Geometry: final body of the model. Coordinates: model frame, mm. A direction names the side the tool comes from. Give positions to 0.01 mm unless a question says otherwise; leave off trailing zeros. Write each loop counter-clockwise with the first axis right and the second up, starting at its lowest first coordinate (ties: lowest second). Pieces come first, ordered by that corner, then holes. Notation, with made-up numbers: M 24.25,-3.75 L 57.25,-3.75 A13 cw 57.25,11.25 Z; hole C 23.5,3 d9. An arc over 180 degrees is marked long. Use a Markdown table: item, result. Add a question column.
(1) Draft query along X for faces 1 (the flat face through (112, 84, 25)), 2 (the flat face through (54, 0, 25)), 3 (the flat face through (54, 86, -2)). Return one class per face: released by +X, released by -X, zero draft, split by the parting line, or undercut.
(2) Cut plane A-A (y = 70). Output: boundary loops of the cut face in (x, z), plus the area to 3 significant figures.
(3) Cut plane B-B (x = 13.5). Output: boundary loops of the cut face in (y, z), plus the area to 3 significant figures.
(4) Cut plane C-C (z = 11). Output: boundary loops of the cut face in (x, y), plus the area to 3 significant figures.
(5) Reachability of faces 4 (the flat face through (0, 84, 25)), 5 (the cylindrical face through (110.378, 26.419, 31.548)), 6 (the cylindrical face through (24.54, -0.38, 27.95)) from +Z, -Z, +X, -X, +Y, -Y: full face, straight path, thin tool, end or side. Return the list, or none.
(6) Pin query (flat end, axial travel): pin 1 Ø3 at (x, y) = (4.5, 8) entering from -Z; pin 2 Ø7.5 at (x, y) = (80.5, 142.5) entering from +Z; pin 3 Ø4 at (x, y) = (66, 149.5) entering from +Z; pin 4 Ø3.5 at (y, z) = (110, 30) entering from +X. Return the tip coordinate at first contact, or that it passes through.
(7) Material intervals for L1, parallel to X at y = 143, z = 0.5; L2, parallel to Y at x = 70, z = 16; L3, parallel to X at y = 159, z = 24.5, sorted ascending.
(8) Cut plane D-D (y = 25). Output: boundary loops of the cut face in (x, z).
```python
from build123d import *

# Parameters (mm, degrees)
CYLINDER002_R            = 2.1
CYLINDER002_DEPTH        = 10
CYLINDER002_PITCH_ANGLE  = 90
CYLINDER001_R            = 1.6
CYLINDER001_DEPTH        = 7
ARRAY001_X_COUNT         = 2
ARRAY001_X_PITCH         = 76
ARRAY001_Y_COUNT         = 2
ARRAY001_Y_PITCH         = 135
CLONE003_ROLL_ANGLE      = 90
CLONE003_PLACEMENT_ANGLE = -90
CYLINDER_R               = 3.5
CYLINDER_DEPTH           = 3.5
ARRAY_X_COUNT            = 2
ARRAY_X_PITCH            = 76
ARRAY_Y_COUNT            = 2
ARRAY_Y_PITCH            = 135
CONE_PITCH_ANGLE         = -90
CLONE002_ROLL_ANGLE      = -90
CLONE002_PLACEMENT_ANGLE = -90
BOX_W                    = 110
BOX_H                    = 170
BOX_DEPTH                = 50
THICKNESS_T              = 2


with BuildPart() as cylinder002:
    # Cylinder002 → Cylinder002 (new body)
    with BuildSketch(Plane.XY):
        Circle(CYLINDER002_R)
    extrude(amount=CYLINDER002_DEPTH)


with BuildPart() as cylinder002_1:
    # Cylinder002 pitch: moved
    add(cylinder002.part.rotate(Axis((0, 0, 0), (0, 1, 0)), CYLINDER002_PITCH_ANGLE))


with BuildPart() as cylinder002_2:
    # Cylinder002 placement: moved
    add(cylinder002_1.part.moved(Location((108, 25, 30))))


with BuildPart() as clone_of_cylinder002:
    # Clone001 base: copy of Cylinder002
    add(cylinder002_2.part)


with BuildPart() as clone_of_cylinder002_1:
    # Clone001 placement: moved
    add(clone_of_cylinder002.part.moved(Location((0, 85, 0))))


with BuildPart() as mount_holes:
    # Cylinder001 → Cylinder001 (new body)
    with BuildSketch(Plane.XY.offset(-3)):
        Circle(CYLINDER001_R)
    extrude(amount=CYLINDER001_DEPTH)

    # Array001 X: mount_holes ×2


with BuildPart() as mount_holes_1:
    add(mount_holes.part)
    with Locations(*[(i * ARRAY001_X_PITCH, 0, 0) for i in range(1, ARRAY001_X_COUNT)]):
        add(mount_holes.part)

    # Array001 Y: mount_holes ×2


with BuildPart() as mount_holes_2:
    add(mount_holes_1.part)
    with Locations(*[(0, i * ARRAY001_Y_PITCH, 0) for i in range(1, ARRAY001_Y_COUNT)]):
        add(mount_holes_1.part)


with BuildPart() as mount_holes_3:
    # Array001 placement: moved
    add(mount_holes_2.part.moved(Location((4.5, 8, 0))))


with BuildPart() as fusion001:
    # Clone003 base: copy of Cylinder002
    add(cylinder002_2.part)


with BuildPart() as fusion001_1:
    # Clone003 roll: moved
    add(fusion001.part.rotate(Axis((0, 0, 0), (1, 0, 0)), CLONE003_ROLL_ANGLE))


with BuildPart() as fusion001_2:
    # Clone003 placement: moved
    add(fusion001_1.part.moved(Location((55, 113, 5))).rotate(Axis((55, 113, 5), (0, 0, 1)), CLONE003_PLACEMENT_ANGLE))

    # Fusion001: union Clone of Cylinder002, Cylinder002, mount_holes
    add(clone_of_cylinder002_1.part)
    add(cylinder002_2.part)
    add(mount_holes_3.part)


with BuildPart() as mount_points:
    # Cylinder → Cylinder (new body)
    with BuildSketch(Plane.XY):
        Circle(CYLINDER_R)
    extrude(amount=CYLINDER_DEPTH)

    # Array X: mount_points ×2


with BuildPart() as mount_points_1:
    add(mount_points.part)
    with Locations(*[(i * ARRAY_X_PITCH, 0, 0) for i in range(1, ARRAY_X_COUNT)]):
        add(mount_points.part)

    # Array Y: mount_points ×2


with BuildPart() as mount_points_2:
    add(mount_points_1.part)
    with Locations(*[(0, i * ARRAY_Y_PITCH, 0) for i in range(1, ARRAY_Y_COUNT)]):
        add(mount_points_1.part)


with BuildPart() as mount_points_3:
    # Array placement: moved
    add(mount_points_2.part.moved(Location((4.5, 8, 0))))


with BuildPart() as cone:
    # Cone → Cone (revolve)
    with BuildSketch(Plane.XZ):
        Polygon((0, 0), (8, 0), (4, 1.2), (0, 1.2), align=None)
    revolve(axis=Axis((0, 0, 0), (0, 0, 1)))


with BuildPart() as cone_1:
    # Cone pitch: moved
    add(cone.part.rotate(Axis((0, 0, 0), (0, 1, 0)), CONE_PITCH_ANGLE))


with BuildPart() as cone_2:
    # Cone placement: moved
    add(cone_1.part.moved(Location((110, 25, 30))))


with BuildPart() as clone_of_cone:
    # Clone base: copy of Cone
    add(cone_2.part)


with BuildPart() as clone_of_cone_1:
    # Clone placement: moved
    add(clone_of_cone.part.moved(Location((0, 85, 0))))


with BuildPart() as clone_of_cone001:
    # Clone002 base: copy of Cone
    add(cone_2.part)


with BuildPart() as clone_of_cone001_1:
    # Clone002 roll: moved
    add(clone_of_cone001.part.rotate(Axis((0, 0, 0), (1, 0, 0)), CLONE002_ROLL_ANGLE))


with BuildPart() as clone_of_cone001_2:
    # Clone002 placement: moved
    add(clone_of_cone001_1.part.moved(Location((-5, 110, 55))).rotate(Axis((-5, 110, 55), (0, 0, 1)), CLONE002_PLACEMENT_ANGLE))


with BuildPart() as case_with_mount_holes:
    # Box → Box (new body)
    with BuildSketch(Plane.XY):
        with Locations((55, 85)):
            Rectangle(BOX_W, BOX_H)
    extrude(amount=BOX_DEPTH)

    # Thickness
    thickness_openings = [case_with_mount_holes.faces().sort_by_distance(p)[0] for p in [
        (55, 85, 50),
    ]]
    offset(amount=THICKNESS_T, openings=thickness_openings)

    # Fusion: union mount_points, Clone of Cone, Cone, Clone of Cone001
    add(mount_points_3.part)
    add(clone_of_cone_1.part)
    add(cone_2.part)
    add(clone_of_cone001_2.part)

    # Cut: cut Fusion001
    add(fusion001_2.part, mode=Mode.SUBTRACT)


solid = case_with_mount_holes.part
```
Answer list:
| question | item | result |
|---|---|---|
| 1 | face 1 | released by +X |
| 1 | face 2 | undercut |
| 1 | face 3 | zero draft |
| 2 | outline | M -2,0 A2 ccw 0,-2 L 110,-2 A2 ccw 112,0 L 112,50 L 110,50 L 110,0 L 0,0 L 0,50 L -2,50 Z |
| 2 | area | 426 mm² |
| 3 | outline | M -2,0 A2 ccw 0,-2 L 170,-2 A2 ccw 172,0 L 172,50 L 170,50 L 170,0 L 0,0 L 0,50 L -2,50 Z |
| 3 | area | 546 mm² |
| 4 | outline | M -2,0 A2 ccw 0,-2 L 110,-2 A2 ccw 112,0 L 112,170 A2 ccw 110,172 L 0,172 A2 ccw -2,170 Z; hole M 0,0 L 110,0 L 110,170 L 0,170 Z |
| 4 | area | 1,130 mm² |
| 5 | face 4 | +Z |
| 5 | face 5 | +X |
| 5 | face 6 | -Y |
| 6 | pin 1 | through |
| 6 | pin 2 | z = 3.5 |
| 6 | pin 3 | z = 0 |
| 6 | pin 4 | x = 0 |
| 7 | L1 | -2 to 0, 1 to 2.9, 6.1 to 8, 77 to 78.9, 82.1 to 84, 110 to 112 |
| 7 | L2 | -2 to 0, 170 to 172 |
| 7 | L3 | -2 to 0, 110 to 112 |
| 8 | outline | M -2,0 A2 ccw 0,-2 L 110,-2 A2 ccw 112,0 L 112,27.9 L 108.8,27.9 L 108.8,26 L 110,22 L 110,0 L 0,0 L 0,50 L -2,50 Z; M 108.8,32.1 L 112,32.1 L 112,50 L 110,50 L 110,38 L 108.8,34 Z |
